Design review of the part built by this model. Coordinates are the model's own, in mm. Give positions to 0.01 mm unless a question says otherwise; leave off trailing zeros. Write each loop counter-clockwise with the first axis right and the second up, starting at its lowest first coordinate (ties: lowest second). Pieces come first, ordered by that corner, then holes. Notation, with made-up numbers: M -32,50 L 26,50 A7 cw 26,54 Z; hole C -34.5,-17 d7. An arc over 180 degrees is marked long. One line per item, written item: value. Start each with the question number.
Autodesk Inventor part; units mm, degrees
ref_plane "Start plane" through (0, 0, 12.0828) normal (0, 0, 1) x (1, 0, 0)
ref_plane "End plane" through (0, 0, 387.9172) normal (0, 0, 1) x (1, 0, 0)
ref_plane "Work Plane4" through (-155.3012, 0, -34.0963) normal (0.3162, 0, -0.9487) x (-0.9487, 0, -0.3162)
ref_plane "Start plane" through (0, 0, 12.0828) normal (0, 0, 1) x (1, 0, 0)
ref_plane "End plane" through (0, 0, 387.9172) normal (0, 0, 1) x (1, 0, 0)
sketch "Sketch" plane through (0, 0, 0) normal (0, 0, 1) x (1, 0, 0)
  circle A0 centre (0, 0) radius 13.3858
  circle A1 centre (0, 0) radius 16.764
  dimension "d0" = 33.528
  dimension "d1" = 3.3782
extrude "Body" add sketch "Sketch" along normal up to surface (375.8344 mm away) from surface at 12.0828
sketch "Sketch3" plane through (0, 0, 0) normal (0, 0, 1) x (1, 0, 0)
  line L0 (0, 0) -> (10, 0)
ref_plane "Work Plane3" through (0, 0, 0) normal (0, -1, 0) x (1, 0, 0)
ref_plane "Work Plane4" through (-155.3012, 0, -34.0963) normal (0.3162, 0, -0.9487) x (-0.9487, 0, -0.3162)
split "Split1" plane through (-155.3012, 0, -34.0963) removes the side toward (0.3162, 0, -0.9487)
ref_plane "Work Plane5" through (-5.3012, 0, 384.0963) normal (0.3162, 0, 0.9487) x (0.9487, 0, -0.3162)
split "Split2" plane through (-5.3012, 0, 384.0963) removes the side toward (0.3162, 0, 0.9487)
sketch "Sketch4" plane through (0, 0, 0) normal (0, -1, 0) x (1, 0, 0)
  line L0 (-2, 12.0828) -> (12, 12.0828)
  line L1 (-2, 387.9172) -> (12, 387.9172)
  dimension "d7" = 375.8344
equation "\"d0\" = G_H"
equation "\"d1\" = G_T"
equation "\"d2\" = G_L"
equation "\"G_H\" = 33.528"
equation "\"G_T\" = 3.3782"
equation "\"G_L\" = d7"
equation "\"G_OFFSET_START\" = -12.08281"
equation "\"G_OFFSET_END\" = -12.08281"
equation "\"d4\" = -G_OFFSET_START"
equation "\"d5\" = G_OFFSET_END + B_L"
equation "\"B_L\" = 400"
properties part number "ANSI - 1 x 0.133 - 14.797" material "Steel, Mild"
Q1. Take a section at C-C, the plane z = 225.5. Give the boundary of the cut face in (x, y).
Q2. Take a section at B-B, the plane y = 9. Give the boundary of the cut face in (x, z), then the cut area to 3 significant figures.
Q3. For P1, Ø12, axis at x = -13.5, y = 3.5, coming from the -Z side; P2, Ø1.5, axis at x = 13.5, y = -1.5, coming from the -Z side; P3, Ø3, axis at x = 10, y = -10, coming from the -Z side; P4, Ø6, axis at x = -9, z = 276.5, coming from the +Y side, all flat-tipped, find the tip position at first contact; note any pin that passes through.
Q4. The part is to be moulded in two halves that separate along X. For faces 1 (the face through (1.164, -13.738, 381.942)), 2 (the face through (16, -5, 197)), 3 (the face through (6.177, 11.876, 197.381)), say which applies: pulls with the +X half, pulls with the -X half, needs draft (parallel to the pull), parting line crosses it, or undercut.
Q5. Take a section at A-A, the plane x = -8.5. Give the boundary of the cut face in (y, z).
Q6. Wall thickness on line 1 (X direction, y = 0, z = 274.5); line 2 (Y direction, x = 1.5, z = 203.5): over which ranges is each line inside the solid? List them lowest first. Write a range as from..to.
Results list:
1. outline: C 0,0 d33.53; hole C 0,0 d26.77
2. outline: M -14.14,12.95 L -9.91,14.36 L -9.91,385.63 L -14.14,387.04 Z; M 9.91,20.97 L 14.14,22.38 L 14.14,377.62 L 9.91,379.03 Z
2. area: 3,090 mm^2
3. P1: stops at z = 12.08
3. P2: stops at z = 22.07
3. P3: stops at z = 20.51
3. P4: stops at y = 15.65
4. face 1: pulls with the +X half
4. face 2: parting line crosses it
4. face 3: undercut
5. outline: M -14.45,14.83 L -10.34,14.83 L -10.34,385.16 L -14.45,385.16 Z; M 10.34,14.83 L 14.45,14.83 L 14.45,385.16 L 10.34,385.16 Z
6. line 1: x = -16.76..-13.39, 13.39..16.76
6. line 2: y = -16.7..-13.3, 13.3..16.7
